Here's the drawing with two shaded views (mm, measured from the low corner). I have some questions. A direction names the side the tool comes from. Coordinates: 2 decimals unless noted, no trailing zeros. Write each loop counter-clockwise with the first axis right and the second up, starting at its lowest first coordinate (ties: lowest second). Pieces come first, ordered by that corner, then holes.
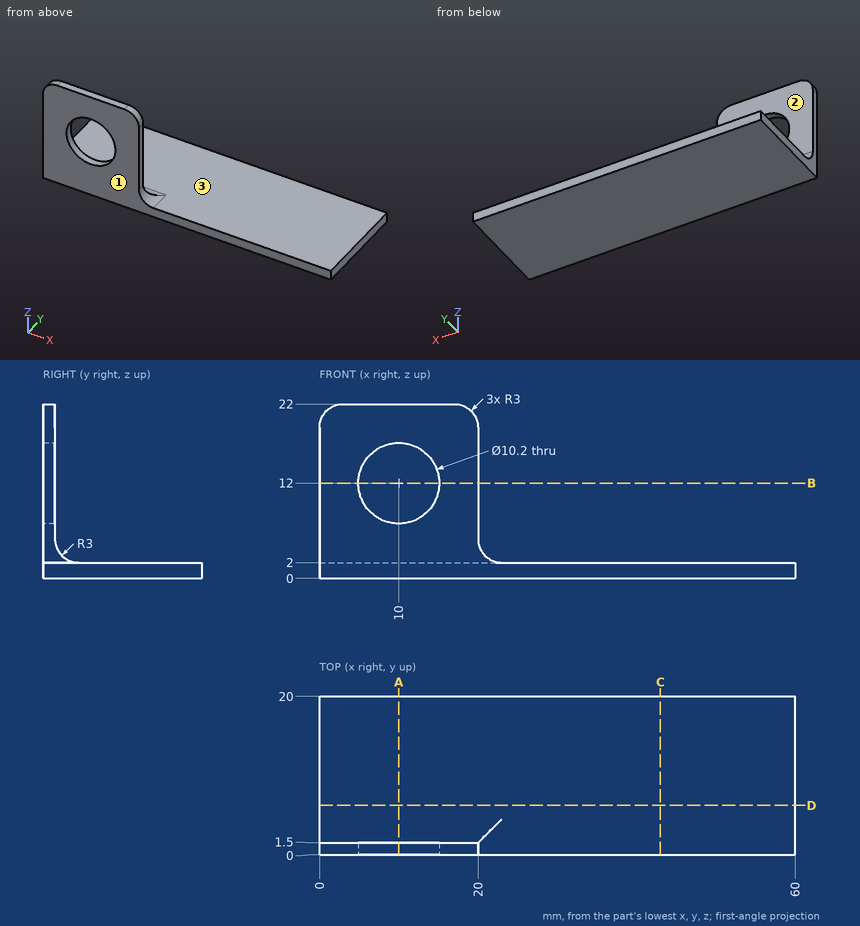
1. Please list where these lines run through material, in increasing order: line 1 along X through (y, z) = (0.9, 12); line 2 along Z through (x, y) = (12, 11.5); line 3 along Y through (x, z) = (4.5, 6.25).
Verdict:
line 1: x = 0 to 4.9, 15.1 to 20
line 2: z = 0 to 2
line 3: y = 0 to 1.5
2. I want a section at A-A on x = 10. Please give me the cut outline in (y, z), plus the area to 3 significant figures.
Verdict:
outline: (0, 0) - (20, 0) - (20, 2) - (4.5, 2) arc R3 cw to (1.5, 5) - (1.5, 6.9) - (0, 6.9) - close; (0, 17.1) - (1.5, 17.1) - (1.5, 22) - (0, 22) - close
area: 56.6 mm2
3. I want a section at D-D on y = 6.25. Please give me the cut outline in (x, z).
Verdict:
outline: (0, 0) - (60, 0) - (60, 2) - (0, 2) - close
4. On a 3-axis mill with a long thin cutter (end or side, diameter ignored), from which of +Z, -Z, +X, -X, +Y, -Y can I reach the whole of each face in a straight line? I mean the marked faces 1, 2 and 3. Say none if no direction works.
Verdict:
face 1: +Z, -Z, +X, -X, -Y
face 2: +Z, +X, -X, +Y
face 3: +Z, +X, +Y
5. I want a section at B-B on z = 12. Please give me the cut outline in (x, y).
Verdict:
outline: (0, 0) - (4.9, 0) - (4.9, 1.5) - (0, 1.5) - close; (15.1, 0) - (20, 0) - (20, 1.5) - (15.1, 1.5) - close
6. For pin 1 (12 mm diameter, centred on x = 47, y = 11.5, fed in from -Z); pin 2 (6 mm diameter, centred on x = 28.5, y = 5, fed in from +Z); pin 3 (1.2 mm diameter, centred on y = 1, z = 12.5, fed in from +X), each with a flat end and sliding along its axis, tell me the tip position at first contact or that it passes through.
Verdict:
pin 1: stops at z = 0
pin 2: stops at z = 2
pin 3: stops at x = 20
7. I want a section at C-C on x = 43. Please give me the cut outline in (y, z), plus the area to 3 significant figures.
Verdict:
outline: (0, 0) - (20, 0) - (20, 2) - (0, 2) - close
area: 40.0 mm2
